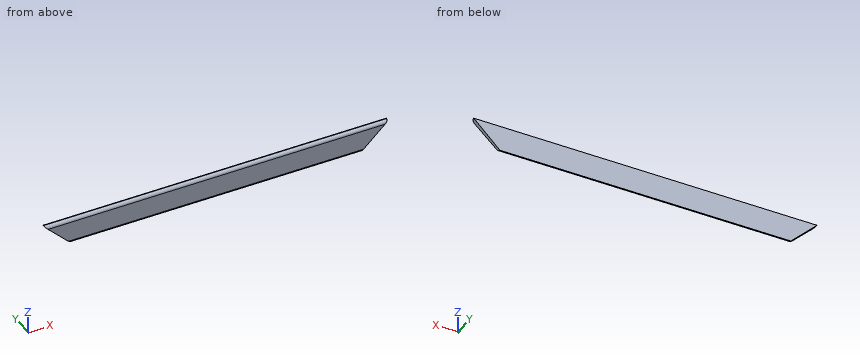
from build123d import *

# Parameters (mm, degrees)
EXTRUDE039434_DEPTH = 500


with BuildPart() as extrude039434_internal_superior:
    # Sketch223 (on Sketch) → Extrude039434 (new body, symmetric)
    with BuildSketch(Plane.XZ):
        Polygon((-600, 2300), (600, 2300), (200, 1900), (-200, 1900), align=None)
    extrude(amount=EXTRUDE039434_DEPTH, both=True)


with BuildPart() as external_trim_horizontal:
    # Sweep011: sweep along a path in Sketch194
    with BuildLine(Plane.XZ.offset(140)) as sweep011_path:
        Line((-390, 2090), (-390, 0))
        Line((-390, 0), (390, 0))
        Line((390, 0), (390, 2090))
        Line((390, 2090), (-390, 2090))
    # Clone2D027 (on Sketch) → Sweep011 (sweep)
    with BuildSketch(Plane(origin=(0, -140, 0), x_dir=(0, 0, 1), z_dir=(1, 0, 0))):
        with BuildLine():
            Line((-61.571224, 10), (-5.678418, 7))
            ThreePointArc((-5.678418, 7), (-1.645147, 5.136003), (0, 1.008624))
            Line((0, 1.008624), (0, 0))
            Line((0, 0), (-70, 0))
            Line((-70, 0), (-70, 2.011499))
            ThreePointArc((-70, 2.011499), (-67.503171, 7.81797), (-61.571224, 10))
        make_face()
    sweep(path=sweep011_path.line, is_frenet=True, transition=Transition.RIGHT)

    # Common: intersect Extrude039434_Internal_superior_
    add(extrude039434_internal_superior.part, mode=Mode.INTERSECT)


solid = external_trim_horizontal.part
Design review of the part built by this model. Coordinates are the model's own, in mm. Coordinates: 2 decimals unless noted, no trailing zeros. Order: outer loops, then holes, each group sorted by start corner. A loop starts at its lowest first (then second) coordinate and runs counter-clockwise, first axis right, second up.
Item 1: For pin 1 Ø1.5 at (y, z) = (-144.5, 2129) entering from +X; pin 2 Ø3 at (x, z) = (-104.5, 2112.5) entering from -Y; pin 3 Ø1.5 at (x, y) = (74.5, -148) entering from +Z, all flat-tipped, find the tip position at first contact; note any pin that passes through.
Item 2: Take a section at A-A, the plane x = 269. Write out the cut boundary in (y, z), then the cut area to 3 significant figures.
Item 3: For line 1 (Y direction, x = -181.5, z = 2099); line 2 (Y direction, x = 371.5, z = 2095); line 3 (Z direction, x = -86, y = -143.5), list the stretches that pass through material, from the lowest coordinate up.
Item 4: Take a section at C-C, the plane y = -145. Write out the cut boundary in (x, z).
Item 5: Take a section at B-B, the plane z = 2142. Write out the cut boundary in (x, y), then the cut area to 3 significant figures.
The answers:
1. pin 1: stops at x = 429.75
1. pin 2: stops at y = -147.98
1. pin 3: stops at z = 2158.05
2. outline: (-150, 2151.57) - (-147, 2095.68) arc R6 ccw to (-141.01, 2090) - (-140, 2090) - (-140, 2160) - (-142.01, 2160) arc R8 ccw to start
2. area: 578 mm2
3. line 1: y = -147.18 to -140
3. line 2: y = -146.92 to -140
3. line 3: z = 2090.54 to 2159.86
4. outline: (-459.42, 2159.42) - (-391.52, 2091.52) - (391.52, 2091.52) - (459.42, 2159.42) - close
5. outline: (-442, -149.49) - (442, -149.49) - (442, -140) - (-442, -140) - close
5. area: 8,390 mm2
